Source: CAD feature listing. Evaluate the final solid. Frame: model axes, mm. Face numbers are marked on the shaded views. A direction names the side the tool comes from. Give positions to 0.01 mm unless a question says otherwise; leave off trailing zeros. Loops run counter-clockwise (first coordinate to the right, second up) from the corner with the lowest first, then second, coordinate; pieces in that order, holes last.
```python
from build123d import *

# Parameters (mm, degrees)
SKETCH_1_W            = 15
SKETCH_1_H            = 38
EXTRUDE_1_DEPTH       = 3
EXTRUDE_4_DEPTH       = 3
SKETCH_6_W            = 10
SKETCH_6_H            = 2.5
EXTRUDE_5_DEPTH       = 9
HOLE_WIZARD_3_0_3_1_D = 3
FILLET_1_R            = 4


with BuildPart() as part:
    # 스케치1 → 보스-돌출1 (new body)
    with BuildSketch(Plane.XY):
        Rectangle(SKETCH_1_W, SKETCH_1_H)
    extrude(amount=EXTRUDE_1_DEPTH)

    # 스케치5 → 보스-돌출4 (add)
    with BuildSketch(Plane(origin=(0, 0, 0), x_dir=(-1, 0, 0), z_dir=(0, 0, -1))):
        Polygon((-7.5, 16.5), (-10.5, 16.5), (-10.5, 18.5), (-13.5, 18.5), (-13.5, 10.5), (-10.5, 10.5), (-10.5, 12.5), (-7.5, 12.5), align=None)
        Polygon((7.5, 16.5), (7.5, 12.5), (10.5, 12.5), (10.5, 10.5), (13.5, 10.5), (13.5, 18.5), (10.5, 18.5), (10.5, 16.5), align=None)
        Polygon((7.5, -16.5), (10.5, -16.5), (10.5, -18.5), (13.5, -18.5), (13.5, -10.5), (10.5, -10.5), (10.5, -12.5), (7.5, -12.5), align=None)
        Polygon((-7.5, -16.5), (-7.5, -12.5), (-10.5, -12.5), (-10.5, -10.5), (-13.5, -10.5), (-13.5, -18.5), (-10.5, -18.5), (-10.5, -16.5), align=None)
    extrude(amount=-EXTRUDE_4_DEPTH)

    # 스케치6 → 보스-돌출5 (add)
    with BuildSketch(Plane(origin=(0, 0, 0), x_dir=(-1, 0, 0), z_dir=(0, 0, -1))):
        with Locations((0, 17.75)):
            Rectangle(SKETCH_6_W, SKETCH_6_H)
        with Locations((0, -17.75)):
            Rectangle(SKETCH_6_W, SKETCH_6_H)
    extrude(amount=EXTRUDE_5_DEPTH)

    # Ø3.0 (3) 지름 구멍1 (through all)
    with Locations(Plane(origin=(0, 19, 0), x_dir=(1, 0, 0), z_dir=(0, 1, 0))):
        with Locations((0, 6)):
            Hole(HOLE_WIZARD_3_0_3_1_D / 2)

    # 필렛1
    fillet_1_edges = [part.edges().sort_by_distance(p)[0] for p in [
        (5, 17.75, -9),
        (-5, 17.75, -9),
        (-5, -17.75, -9),
        (5, -17.75, -9),
    ]]
    fillet(fillet_1_edges, radius=FILLET_1_R)


solid = part.part
```
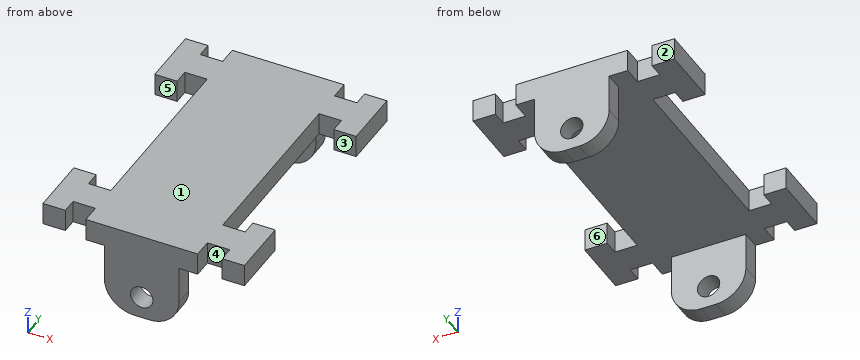
(1) Section B-B, the plane z = -3.25. Return the cut outline in (x, y).
A:
outline: (-5, -19) - (5, -19) - (5, -16.5) - (-5, -16.5) - close; (-5, 16.5) - (5, 16.5) - (5, 19) - (-5, 19) - close
(2) Mould query, pull axis Y, two halves, no side actions, for the marked faces 1, 2 and 3. Classes: pulls with the +Y half, pulls with the -Y half, needs draft (parallel to the pull), parting line crosses it, or undercut.
A:
face 1: needs draft
face 2: pulls with the +Y half
face 3: undercut
(3) Section C-C, the plane x = 0. Return the cut outline in (y, z), then the cut area to 3 significant figures.
A:
outline: (-19, -9) - (-16.5, -9) - (-16.5, -7.5) - (-19, -7.5) - close; (-19, -4.5) - (-16.5, -4.5) - (-16.5, 0) - (16.5, 0) - (16.5, -4.5) - (19, -4.5) - (19, 3) - (-19, 3) - close; (16.5, -9) - (19, -9) - (19, -7.5) - (16.5, -7.5) - close
area: 144 mm2
(4) First-contact query: pin 1 (2.5 mm diameter, centred on x = -12, z = 2, fed in from +Y); pin 2 (4 mm diameter, centred on x = 0, z = -6, fed in from -Y); pin 3 (1.5 mm diameter, centred on x = 8.5, z = 2, fed in from -Y); pin 4 (3.5 mm diameter, centred on y = -4.5, z = 1.5, fed in from +X). Flat tips, straight axial feed; report the tip coordinate or a pass-through.
A:
pin 1: stops at y = 18.5
pin 2: stops at y = -19
pin 3: stops at y = -16.5
pin 4: stops at x = 7.5
(5) Section A-A, the plane x = 11.5. Return the cut outline in (y, z), then the cut area to 3 significant figures.
A:
outline: (-18.5, 0) - (-10.5, 0) - (-10.5, 3) - (-18.5, 3) - close; (10.5, 0) - (18.5, 0) - (18.5, 3) - (10.5, 3) - close
area: 48.0 mm2
(6) Ray query, line 1 along Y through (x, z) = (4.75, -5.5); line 2 along Z through (x, y) = (0, 17.45); line 3 along Y through (x, z) = (-7.75, 2). Return the intervals inside material, ascending.
A:
line 1: y = -19 to -16.5, 16.5 to 19
line 2: z = -9 to -7.5, -4.5 to 3
line 3: y = -16.5 to -12.5, 12.5 to 16.5
(7) Reachability of the marked faces 4, 5 and 6 from +Z, -Z, +X, -X, +Y, -Y: full face, straight path, thin tool, end or side. Return the list, or none.
A:
face 4: +Z, -Z, -Y
face 5: +Z, -Z, -X
face 6: +Z, -Z, +X
(8) Section D-D, the plane z = -6. Return the cut outline in (x, y), then the cut area to 3 significant figures.
A:
outline: (-4.87, -19) - (-1.5, -19) - (-1.5, -16.5) - (-4.87, -16.5) - close; (-4.87, 16.5) - (-1.5, 16.5) - (-1.5, 19) - (-4.87, 19) - close; (1.5, -19) - (4.87, -19) - (4.87, -16.5) - (1.5, -16.5) - close; (1.5, 16.5) - (4.87, 16.5) - (4.87, 19) - (1.5, 19) - close
area: 33.7 mm2
